from build123d import *

# Parameters (mm, degrees)
CROQUIS1_W                 = 100
CROQUIS1_H                 = 150
SALIENTE_EXTRUIR2_DEPTH    = 3
CORTAR_EXTRUIR1_DEPTH      = 91.188691087
CORTAR_EXTRUIR1_DEPTH_BACK = 91.188691087
CROQUIS2_W                 = 15
CROQUIS2_H                 = 100
REDONDEO1_R                = 3


with BuildPart() as part:
    # Croquis1 → Saliente-Extruir2 (new body)
    with BuildSketch(Plane(origin=(0, 0, 0), x_dir=(1, 0, 0), z_dir=(0, 1, 0))):
        Rectangle(CROQUIS1_W, CROQUIS1_H)
    extrude(amount=SALIENTE_EXTRUIR2_DEPTH)

    # Croquis2 → Cortar-Extruir1 (cut, two sides: drawn at the far end of the back side and taken through both)
    with BuildSketch(Plane(origin=(0, 3, 0), x_dir=(1, 0, 0), z_dir=(0, 1, 0)).offset(-CORTAR_EXTRUIR1_DEPTH_BACK)):
        with Locations((-42.5, -25)):
            Rectangle(CROQUIS2_W, CROQUIS2_H)
        with Locations((42.5, -25)):
            Rectangle(CROQUIS2_W, CROQUIS2_H)
    extrude(amount=CORTAR_EXTRUIR1_DEPTH + CORTAR_EXTRUIR1_DEPTH_BACK, mode=Mode.SUBTRACT)

    # Redondeo1
    redondeo1_edges = [part.edges().sort_by_distance(p)[0] for p in [
        (-50, 1.5, -25),
        (-35, 1.5, 75),
        (50, 1.5, -25),
        (35, 1.5, 75),
        (-50, 1.5, -75),
        (50, 1.5, -75),
    ]]
    fillet(redondeo1_edges, radius=REDONDEO1_R)


solid = part.part
Here's how the part is built. I have some questions about the finished solid (model axes, mm). A direction names the side the tool comes from. Give positions to 0.01 mm unless a question says otherwise; leave off trailing zeros. Write each loop counter-clockwise with the first axis right and the second up, starting at its lowest first coordinate (ties: lowest second). Pieces come first, ordered by that corner, then holes. Notation, with made-up numbers: (-17.5, 49) -> (36.5, 49) arc R18 ccw to (36.5, 78) -> close; hole circle Ø7 at (48.5, 22.25). An arc over 180 degrees is marked (long way). Use one line per item in the form item = value. Start each with the question number.
1. Will these pins go through, and if not, where does the flat tip stop? pin 1 Ø1.5 at (y, z) = (1, 17.5) entering from -X; pin 2 Ø1.5 at (y, z) = (1, 34.5) entering from +X; pin 3 Ø0.9 at (x, y) = (-44, 1.5) entering from +Z.
2. Imagine slicing it at B-B on z = 37. List the corners of the cut face in (x, y) for me, plus the area to 3 significant figures.
3. On a 3-axis mill with a long thin cutter (end or side, diameter ignored), from which of +Z, -Z, +X, -X, +Y, -Y can I reach the whole of each face in a straight line? I mean faces 1 (the face through (-49.14, 1.52, -74.1)), 2 (the face through (41, 1, -25)), 3 (the face through (-35, 1, 24)). Say none if no direction works.
4. If I drill on L1, parallel to X at y = 1.5, z = -10; L2, parallel to Z at x = 39, y = 1.5; L3, parallel to Z at x = 33.5, y = 1.35, over which ranges is the centre line in solid material (lowest first)?
5. Imagine slicing it at A-A on y = 1.25. List the corners of the cut face in (x, z) for me.
Entries:
q1.pin_1 = -35
q1.pin_2 = 35
q1.pin_3 = -25
q2.outline = (-35, 0) -> (35, 0) -> (35, 3) -> (-35, 3) -> close
q2.area = 210 mm²
q3.face_1 = -Z, -X, +Y, -Y
q3.face_2 = +Z, +X, +Y, -Y
q3.face_3 = +Z, -X, +Y, -Y
q4.L1 = -35 to 35
q4.L2 = -75 to -25
q4.L3 = -75 to 74.6
q5.outline = (-50, -72) arc R3 ccw to (-47, -75) -> (47, -75) arc R3 ccw to (50, -72) -> (50, -28) arc R3 ccw to (47, -25) -> (35, -25) -> (35, 72) arc R3 ccw to (32, 75) -> (-32, 75) arc R3 ccw to (-35, 72) -> (-35, -25) -> (-47, -25) arc R3 ccw to (-50, -28) -> close
